Solid Edge part; units mm, degrees
sketch "Sketch1" plane through (0, 0, 0) normal (0, 0, 1) x (1, 0, 0)
  line L0 (-67.5, -22.5) -> (67.5, -22.5)
  line L1 (67.5, -22.5) -> (67.5, 22.5)
  line L2 (67.5, 22.5) -> (-67.5, 22.5)
  line L3 (-67.5, 22.5) -> (-67.5, -22.5)
  circle A0 centre (-45, 0) radius 10
  circle A1 centre (45, 0) radius 10
extrude "Protrusion1" add sketch "Sketch1" along normal blind 10
fillet "Round_1" radius 22.5 4 edges at (67.5, -22.5, 5) (67.5, 22.5, 5) (-67.5, -22.5, 5) (-67.5, 22.5, 5)
sketch "Sketch2" plane through (0, 22.5, 5) normal (0, 1, 0) x (1, 0, 0)
  line L0 (-15, 60) -> (15, 60)
  line L1 (15, 60) -> (24.5, 5)
  line L2 (-24.5, 5) -> (24.5, 5)
  line L3 (-15, 60) -> (-24.5, 5)
extrude "ExtrudedProtrusion_2" add sketch "Sketch2" against normal blind 22.5
sketch "Sketch3" plane through (0, 10, 0) normal (0, -1, 0) x (1, 0, 0)
  line L0 (15, -85) -> (-15, -85)
  line L1 (-15, -85) -> (-15, -55)
  line L2 (-15, -55) -> (15, -55)
  line L3 (15, -85) -> (15, -55)
  line L4 (10, -60.5862) -> (10, -80.5862)
  line L5 (10, -80.5862) -> (-10, -80.5862)
  line L6 (-10, -80.5862) -> (-10, -60.5862)
  line L7 (-10, -60.5862) -> (10, -60.5862)
extrude "ExtrudedProtrusion_4" add sketch "Sketch3" against normal blind 12.5
sketch "Sketch4" plane through (0, 10, 0) normal (0, -1, 0) x (1, 0, 0)
  line L0 (15, -55) -> (15, -85)
  line L1 (15, -85) -> (-15, -85)
  line L2 (-15, -85) -> (-15, -55)
  line L3 (-15, -55) -> (15, -55)
  line L4 (10, -80.5862) -> (-10, -80.5862)
  line L5 (-10, -80.5862) -> (-10, -60.5862)
  line L6 (-10, -60.5862) -> (10, -60.5862)
  line L7 (10, -60.5862) -> (10, -80.5862)
extrude "ExtrudedProtrusion_5" add sketch "Sketch4" along normal blind 17.5
sketch "Sketch5" plane through (0, 2.5, -70) normal (0, -1, 0) x (-1, 0, 0)
  line L0 (-18, 12) -> (-40, 12)
  line L1 (-40, -12) -> (-18, -12)
  arc A0 (-18, -12) -> (-15, -15) centre (-18, -15) cw
  line L2 (-15, 15) -> (-15, -15)
  arc A1 (-18, 12) -> (-15, 15) centre (-18, 15) ccw
  arc A2 (-40, -12) -> (-40, 12) centre (-40, 0) cw
  circle A3 centre (-40, 0) radius 5
  line L3 (40, 12) -> (18, 12)
  arc A4 (15, 15) -> (18, 12) centre (18, 15) ccw
  line L4 (15, 15) -> (15, -15)
  arc A5 (15, -15) -> (18, -12) centre (18, -15) cw
  line L5 (40, -12) -> (18, -12)
  arc A6 (40, 12) -> (40, -12) centre (40, 0) cw
  circle A7 centre (40, 0) radius 5
extrude "ExtrudedProtrusion_7" add sketch "Sketch5" against normal blind 10
sketch "Sketch6" plane through (7.5, 0, 0) normal (1, 0, 0) x (0, 1, 0)
  line L0 (0, 0) -> (-22.5, 0)
  line L1 (-22.5, 0) -> (-7.5, -55)
  line L2 (-7.5, -55) -> (0, -55)
  line L3 (0, -55) -> (0, 0)
extrude "ExtrudedProtrusion_8" add sketch "Sketch6" against normal blind 15
Source: CAD feature listing. Evaluate the final solid. Frame: model axes, mm. A direction names the side the tool comes from. Round coordinates to 2 decimals unless told otherwise and drop trailing zeros. Loops run counter-clockwise (first coordinate to the right, second up) from the corner with the lowest first, then second, coordinate; pieces in that order, holes last. Notation, with made-up numbers: (64.25, 26.5) - (103.25, 26.5) arc R33 cw to (103.25, 56.5) - close; hole circle Ø7 at (71, -6). An arc over 180 degrees is marked (long way). Write item = value, one per line. Start each with the question number.
(1) Ray query, line 1 along X through (y, z) = (7.5, -70); line 2 along Z through (x, y) = (40, 10); line 3 along Z through (x, y) = (-40, 7). Return the intervals inside material, ascending. Write a range as from..to.
(2) Section query D-D, the plane y = -18.5. Output: boundary loops of the cut face in (x, z).
(3) Pin query (flat end, axial travel): pin 1 (6 mm diameter, centred on x = 40.5, z = -71, fed in from -Y); pin 2 (15 mm diameter, centred on x = 36, z = -67, fed in from +Y); pin 3 (8 mm diameter, centred on y = -2.5, z = -66.5, fed in from -X); pin 4 (10 mm diameter, centred on y = 17, z = -54, fed in from +X). Return the tip coordinate at first contact, or that it passes through.
(4) Section query A-A, the plane z = -70. Output: boundary loops of the cut face in (x, y), plus the area to 3 significant figures.
(5) Set-up query: faces 1 (the face through (0, 7, -60.586)), 2 (the face through (37, -10, 0)), 3 (the face through (19.683, 11.408, -27.885)), 4 (the face through (35, 0, 5)). Return all of +Z, -Z, +X, -X, +Y, -Y with unobstructed straight access to the full face (end or side cutting, diameter ignored); none if empty.
(6) Pull-direction query (Z, two-part tool) for faces 5 (the face through (-1, -22.5, 5)), 6 (the face through (15.9, 7.43, -82.86)), 7 (the face through (-14, 0, -21)); classes: +Z half, -Z half, draft (parallel to the pull), parting line (faces both ways), or undercut.
(7) Section query B-B, the plane y = 4. State how many separate pieces and enclosed holes the cut face has, plus the area to 3 significant figures.
(8) Section query C-C, the plane z = -6. Output: boundary loops of the cut face in (x, y), plus the area to 3 significant figures.
Conclusion:
q1.line_1 = -52..-45, -35..-10, 10..35, 45..52
q1.line_2 = -82..-75, -65..-58, 0..10
q1.line_3 = -82..-75, -65..-58
q2.outline = (-57.81, 0) - (-7.5, 0) - (-7.5, -14.67) - (7.5, -14.67) - (7.5, 0) - (57.81, 0) - (57.81, 10) - (-57.81, 10) - close
q3.pin_1 = through
q3.pin_2 = 12.5
q3.pin_3 = -15
q3.pin_4 = 16.04
q4.outline = (-52, 2.5) - (-45, 2.5) - (-45, 12.5) - (-52, 12.5) - close; (-35, 2.5) - (-15, 2.5) - (-15, -7.5) - (-10, -7.5) - (-10, 22.5) - (-15, 22.5) - (-15, 12.5) - (-35, 12.5) - close; (10, -7.5) - (15, -7.5) - (15, 2.5) - (35, 2.5) - (35, 12.5) - (15, 12.5) - (15, 22.5) - (10, 22.5) - close; (45, 2.5) - (52, 2.5) - (52, 12.5) - (45, 12.5) - close
q4.area = 840 mm2
q5.face_1 = +Y, -Y
q5.face_2 = +X, -Y
q5.face_3 = +X, +Y, -Y
q5.face_4 = +Z
q6.face_5 = draft
q6.face_6 = -Z half
q6.face_7 = undercut
q7.separate_pieces = 3
q7.enclosed_holes = 3
q7.area = 5,150 mm2
q8.outline = (-23.46, 0) - (-7.5, 0) - (-7.5, -20.86) - (7.5, -20.86) - (7.5, 0) - (23.46, 0) - (23.46, 22.5) - (-23.46, 22.5) - close
q8.area = 1,370 mm2
